For this review, take the finished solid that the model builds, in its own axes (mm). A direction names the side the tool comes from. Round coordinates to 2 decimals unless told otherwise and drop trailing zeros. Write each loop counter-clockwise with the first axis right and the second up, starting at its lowest first coordinate (ties: lowest second). Pieces come first, ordered by that corner, then holes. Notation, with made-up numbers: (31.5, 8.25) - (75.5, 8.25) arc R14 ccw to (75.5, 21.25) - close; hole circle Ø8 at (72.5, -28.75). An arc over 180 degrees is marked (long way). One line per item, written item: value. Start each with the question number.
Q1. Add section B-B on y = -138.5. Write out the cut boundary in (x, z), and give its area (3 significant figures).
Q2. For probe 1 along Y at (x, z) = (417, 85); probe 2 along Z at (x, y) = (266, -118); probe 3 along Z at (x, y) = (209, -203), list the stretches that pass through material, from the lowest coordinate up.
Q3. Clearance check with flat-ended pins moving along their axes: pin 1 Ø8 at (x, y) = (304.5, -26.5) entering from +Z; pin 2 Ø1 at (x, z) = (382.5, 70.5) entering from -Y; pin 3 Ø7.5 at (y, z) = (-260, 106.5) entering from -X; pin 4 Ø1.5 at (x, y) = (339.5, -115.5) entering from -Z. State where each tip first meets the part, or that it passes through.
Q4. Add section A-A on x = 213.5. Write out the cut boundary in (y, z), and give its area (3 significant figures).
Q5. Tool access review of faces 5 (the face through (138, -246, 100.085)), 6 (the face through (431.8, -81, 101)), 7 (the face through (130.82, 25.044, 179.233)), 8 (the face through (254, -246, 113)): name each direction out of +Z, -Z, +X, -X, +Y, -Y from which nothing blocks a thin tool from reaching the whole face with its end or side.
Q6. Add section C-C on z = 322.5. Write out the cut boundary in (x, y), and give its area (3 significant figures).
Q7. Add section D-D on x = 91.5. Write out the cut boundary in (y, z).
Q8. Mouldability with a two-part tool opening along Z and no side actions: class faces 1 (the face through (60.82, 25.04, 231.35)), 2 (the face through (108, 50.8, 164)), 3 (the face through (76.2, -81, 103)), 4 (the face through (50, -165.1, 113)) as +Z half, -Z half, draft (parallel to the pull), parting line (faces both ways), or undercut.
```python
from build123d import *

# Parameters (mm, degrees)
F1_DEPTH = 165.1
F2_W     = 177.8
F2_H     = 25.4
F2_W_2   = 50.8
F3_DEPTH = 165.1
F5_DEPTH = 50.8


with BuildPart() as f1:
    # F0 (on Front) → F1 (new body)
    with BuildSketch(Plane.XZ):
        with BuildLine():
            Line((0, 25.4), (0, 0))
            Line((0, 0), (457.2, 0))
            Line((457.2, 0), (457.2, 25.4))
            Line((457.2, 25.4), (431.8, 25.4))
            Line((431.8, 25.4), (431.8, 177.8))
            Line((431.8, 177.8), (107.95, 177.8))
            Line((107.95, 177.8), (107.95, 577.85))
            ThreePointArc((107.95, 577.85), (76.2, 609.6), (44.45, 577.85))
            Line((44.45, 577.85), (44.45, 177.8))
            Line((44.45, 177.8), (76.2, 177.8))
            Line((76.2, 177.8), (76.2, 25.4))
            Line((76.2, 25.4), (0, 25.4))
        make_face()
    extrude(amount=F1_DEPTH)

    # F2 (on face) → F3 (join)
    with BuildSketch(Plane.XZ.offset(165.1)):
        with Locations((165.1, 112.78545)):
            Rectangle(F2_W, F2_H)
        with Locations((50.8, 112.78545)):
            Rectangle(F2_W_2, F2_H)
    extrude(amount=F3_DEPTH)

    # F4 (on face) → F5 (join)
    with BuildSketch(Plane(origin=(0, 0, 0), x_dir=(-1, 0, 0), z_dir=(0, 1, 0))):
        with BuildLine():
            Line((-50.013161, 193.333121), (-55.298633, 186.161049))
            ThreePointArc((-55.298633, 186.161049), (-52.376747, 189.541366), (-50.013161, 193.333121))
        make_face()
        with BuildLine():
            Line((-117.033699, 102.390224), (-55.298633, 186.161049))
            Line((-55.298633, 186.161049), (-50.013161, 193.333121))
            ThreePointArc((-50.013161, 193.333121), (-61.358561, 231.663771), (-100.070771, 221.697747))
            Line((-100.070771, 221.697747), (-162.443357, 135.562881))
            ThreePointArc((-162.443357, 135.562881), (-156.255653, 96.366456), (-117.033699, 102.390224))
        make_face()
    extrude(amount=F5_DEPTH)


solid = f1.part
```
Result set:
1. outline: (0, 0) - (457.2, 0) - (457.2, 25.4) - (431.8, 25.4) - (431.8, 177.8) - (107.95, 177.8) - (107.95, 577.85) arc R31.75 ccw to (44.45, 577.85) - (44.45, 177.8) - (76.2, 177.8) - (76.2, 25.4) - (0, 25.4) - close
1. area: 92,800 mm^2
2. probe 1: y = -165.1 to 0
2. probe 2: z = 0 to 177.8
2. probe 3: z = 100.09 to 125.49
3. pin 1: stops at z = 177.8
3. pin 2: stops at y = -165.1
3. pin 3: stops at x = 25.4
3. pin 4: stops at z = 0
4. outline: (-330.2, 100.09) - (-165.1, 100.09) - (-165.1, 0) - (0, 0) - (0, 177.8) - (-165.1, 177.8) - (-165.1, 125.49) - (-330.2, 125.49) - close
4. area: 33,500 mm^2
5. face 5: -Z, +X, -X, -Y
5. face 6: +Z, +X, +Y, -Y
5. face 7: +Z, +X, +Y
5. face 8: +Z, -Z, +X, -Y
6. outline: (44.45, -165.1) - (107.95, -165.1) - (107.95, 0) - (44.45, 0) - close
6. area: 10,500 mm^2
7. outline: (-330.2, 100.09) - (-165.1, 100.09) - (-165.1, 0) - (0, 0) - (0, 137.04) - (50.8, 137.04) - (50.8, 230.58) - (0, 230.58) - (0, 605.67) - (-165.1, 605.67) - (-165.1, 125.49) - (-330.2, 125.49) - close
8. face 1: parting line
8. face 2: draft
8. face 3: undercut
8. face 4: undercut
